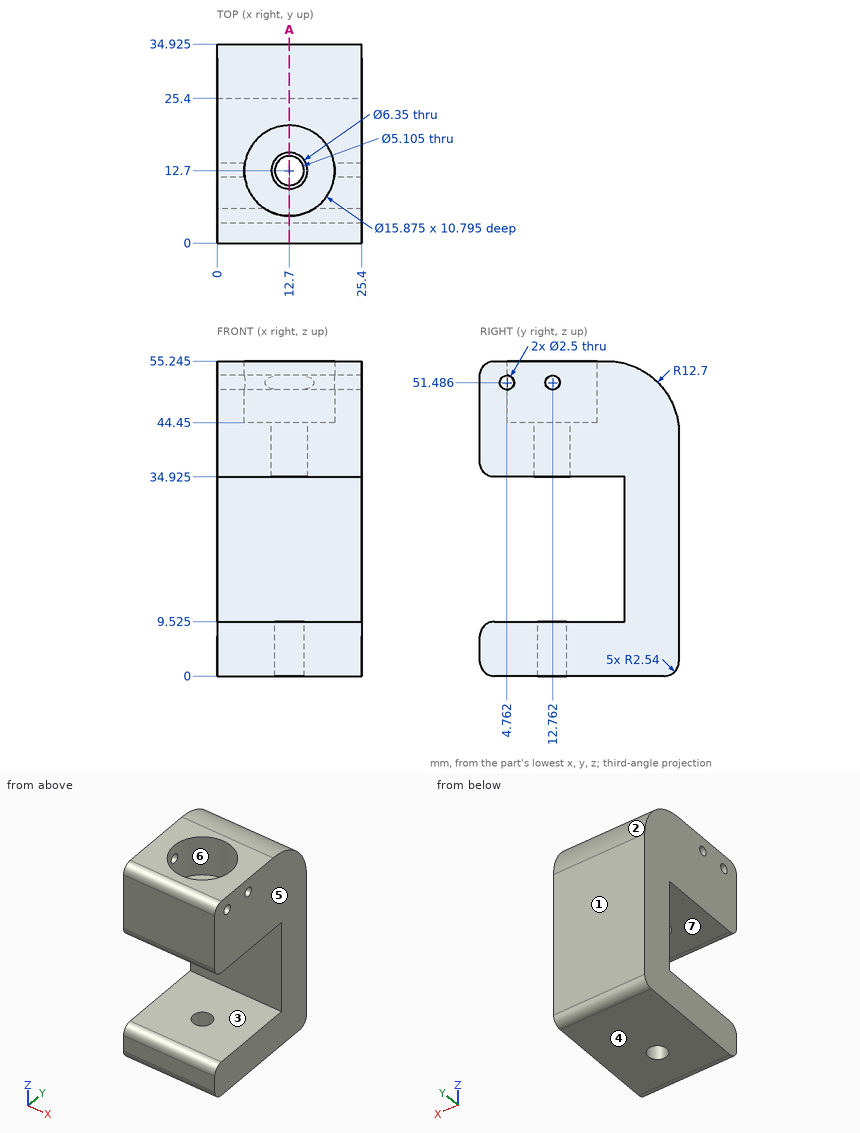
Input: dimensioned drawing with shaded views. Units: mm. Origin: part minimum x, y, z. A direction names the side the tool comes from. Round coordinates to 2 decimals unless told otherwise and drop trailing zeros.
Q1. Pin query (flat end, axial travel): pin 1 (10 mm diameter, centred on x = 9.5, z = 8, fed in from -Y); pin 2 (8.5 mm diameter, centred on x = 12.7, y = 12.7, fed in from +Z); pin 3 (12.5 mm diameter, centred on x = 14, z = 18.5, fed in from -Y); pin 4 (1 mm diameter, centred on x = 11.5, z = 46, fed in from +Y). Return the tip coordinate at first contact, or that it passes through.
Result sheet:
pin 1: stops at y = 0
pin 2: stops at z = 44.45
pin 3: stops at y = 25.4
pin 4: stops at y = 34.58
Q2. Mould query, pull axis Z, two halves, no side actions, for the marked faces 1, 2, 3 and 4. Classes: released by +Z, released by -Z, zero draft, split by the parting line, or undercut.
Result sheet:
face 1: zero draft
face 2: released by +Z
face 3: undercut
face 4: released by -Z
Q3. Section A-A, the plane x = 12.7. Give the number of separate pieces and of enclosed holes in the cut face, and give its area (3 significant figures).
Result sheet:
separate pieces: 3
enclosed holes: 0
area: 960 mm2
Q4. Access query for the marked faces 5, 6 and 7. Directions: +Z, -Z, +X, -X, +Y, -Y. A direction counts if a zero-diameter tool reaches every point of the face in a straight line with its end or side. Return the directions, or none.
Result sheet:
face 5: +Z, -Z, +X, +Y, -Y
face 6: +Z
face 7: +X, -X, -Y
Q5. Material intervals for probe 1 along Z at (x, y) = (17.5, 3) (1 decimal); probe 2 along Y at (x, z) = (12.7, 39) (1 decimal); probe 3 along Y at (x, z) = (14, 12.5) (1 decimal), sorted ascending.
Result sheet:
probe 1: z = 0 to 9.5, 34.9 to 55.2
probe 2: y = 0 to 9.5, 15.9 to 34.9
probe 3: y = 25.4 to 34.9
